Geometry: final body of the model. Coordinates: model frame, mm. Coordinates: 2 decimals unless noted, no trailing zeros. Order: outer loops, then holes, each group sorted by start corner. A loop starts at its lowest first (then second) coordinate and runs counter-clockwise, first axis right, second up. Notation, with made-up numbers: M 9.25,4 L 62.25,4 A10 ccw 62.25,20 Z; hole C -13,-31.75 d8. An arc over 180 degrees is marked long. One line per question, with ' | ' between items.
from build123d import *

# Parameters (mm, degrees)
SKETCH4_R                                         = 4.5339
SKETCH4_R_2                                       = 4.37515
CUT_EXTRUDE2_DEPTH                                = 4.064
CUT_EXTRUDE1_DEPTH                                = 4.064
CIRPATTERN1_COUNT                                 = 14
SKETCH6_R                                         = 1.5875
CUT_EXTRUDE3_DEPTH                                = 12.02520933
CUT_EXTRUDE4_DEPTH                                = 1.016
SKETCH11_R                                        = 6.731
CUT_EXTRUDE6_DEPTH                                = 2.54
SKETCH13_R                                        = 9.525
CUT_EXTRUDE7_DEPTH                                = 12.262802402
BOSS_EXTRUDE2_START                               = -4.064
SKETCH17_R                                        = 1.5875
SKETCH17_R_2                                      = 1.4732
BOSS_EXTRUDE2_DEPTH                               = 4.064
BOSS_EXTRUDE1_START                               = 2.54
SKETCH12_R                                        = 1.4732
BOSS_EXTRUDE1_DEPTH                               = 2.54
CSK_FOR_4_FLAT_HEAD_MACHINE_SCREW_100_D           = 2.9464
CSK_FOR_4_FLAT_HEAD_MACHINE_SCREW_100_CSINK_D     = 6.320409
CSK_FOR_4_FLAT_HEAD_MACHINE_SCREW_100_CSINK_ANGLE = 100


with BuildPart() as part:
    # Sketch1 → Revolve1 (revolve)
    with BuildSketch(Plane.XY, mode=Mode.PRIVATE) as revolve1_sk:
        with BuildLine():
            Line((-5.5626, 1.5875), (5.5626, 1.5875))
            Line((5.5626, 1.5875), (5.5626, 6.731))
            Line((5.5626, 6.731), (5.0419, 6.731))
            ThreePointArc((5.0419, 6.731), (4.654552953, 5.958878742), (4.5212, 5.1054))
            Line((4.5212, 5.1054), (4.5212, 4.5339))
            Line((4.5212, 4.5339), (0.4572, 4.5339))
            Line((0.4572, 4.5339), (0.4572, 5.6769))
            Line((0.4572, 5.6769), (-0.5969, 6.731))
            Line((-0.5969, 6.731), (-5.5626, 6.731))
            Line((-5.5626, 6.731), (-5.5626, 1.5875))
        make_face()
    revolve(revolve1_sk.sketch.rotate(Axis((-5.5626, 0, 0), (1, 0, 0)), 90), axis=Axis((-5.5626, 0, 0), (1, 0, 0)))

    # Sketch4 → Cut-Extrude2 (cut)
    with BuildSketch(Plane(origin=(0.4572, 0, 0), x_dir=(0, 0, -1), z_dir=(1, 0, 0))):
        Circle(SKETCH4_R)
        Circle(SKETCH4_R_2, mode=Mode.SUBTRACT)
    extrude(amount=CUT_EXTRUDE2_DEPTH, mode=Mode.SUBTRACT)

    # Sketch3 → Cut-Extrude1 (cut)
    with BuildSketch(Plane(origin=(0.4572, 0, 0), x_dir=(0, 0, -1), z_dir=(1, 0, 0))):
        with BuildLine():
            Line((-0.641613493, 4.327848154), (-0.345249615, 3.692293767))
            Line((-0.345249615, 3.692293767), (0.345249615, 3.692293767))
            Line((0.345249615, 3.692293767), (0.641613493, 4.327848154))
            ThreePointArc((0.641613493, 4.327848154), (0, 4.37515), (-0.641613493, 4.327848154))
        make_face()
    cut_extrude1 = extrude(amount=CUT_EXTRUDE1_DEPTH, mode=Mode.SUBTRACT)

    # CirPattern1: Cut-Extrude1 ×14 about axis
    cirpattern1_axis = Axis((0, 0, 0), (1, 0, 0))
    for i in range(1, CIRPATTERN1_COUNT):
        add(cut_extrude1.rotate(cirpattern1_axis, i * 360 / CIRPATTERN1_COUNT), mode=Mode.SUBTRACT)

    # Sketch6 → Cut-Extrude3 (cut, through all)
    with BuildSketch(Plane(origin=(0, 0, 0), x_dir=(1, 0, 0), z_dir=(0, 1, 0))):
        with Locations(Location((-2.5527, 0, 0), (0, 0, 90))):
            Circle(SKETCH6_R)
    extrude(amount=CUT_EXTRUDE3_DEPTH, mode=Mode.SUBTRACT)

    # Sketch11 → Cut-Extrude6 (cut)
    with BuildSketch(Plane.ZY.offset(-4.5212)):
        Circle(SKETCH11_R)
    extrude(amount=-CUT_EXTRUDE6_DEPTH, mode=Mode.SUBTRACT)


with BuildPart() as body_2:
    # Sketch7 → Revolve2 (revolve)
    with BuildSketch(Plane.XY, mode=Mode.PRIVATE) as revolve2_sk:
        Polygon((-3.7211, 6.731), (-2.5527, 6.731), (-2.5527, 1.9685), (-3.7211, 1.9685), (-3.9751, 2.2225), (-3.9751, 6.477), align=None)
    revolve(revolve2_sk.sketch.rotate(Axis((-2.5527, 1.9685, 0), (0, 1, 0)), 270), axis=Axis((-2.5527, 1.9685, 0), (0, 1, 0)))

    # Sketch8 → Cut-Extrude4 (cut)
    with BuildSketch(Plane(origin=(0, 6.731, 0), x_dir=(1, 0, 0), z_dir=(0, 1, 0))):
        Polygon((-2.5527, 0.821223023), (-3.2639, 0.410611511), (-3.2639, -0.410611511), (-2.5527, -0.821223023), (-1.8415, -0.410611511), (-1.8415, 0.410611511), align=None)
    extrude(amount=-CUT_EXTRUDE4_DEPTH, mode=Mode.SUBTRACT)


with BuildPart() as cut_extrude7_tool:
    # Sketch13 → Cut-Extrude7 (new, through all)
    with BuildSketch(Plane(origin=(0.4572, 0, 0), x_dir=(0, 0, -1), z_dir=(1, 0, 0))):
        Circle(SKETCH13_R)
    extrude(amount=-CUT_EXTRUDE7_DEPTH)


with BuildPart() as part_1:
    add(part.part)

    # Cut-Extrude7: cut by cut_extrude7_tool
    add(cut_extrude7_tool.part, mode=Mode.SUBTRACT)

    # Sketch17 → Boss-Extrude2 (add)
    with BuildSketch(Plane.ZY.offset(-0.4572).offset(BOSS_EXTRUDE2_START)):
        Circle(SKETCH17_R)
        Circle(SKETCH17_R_2, mode=Mode.SUBTRACT)
    extrude(amount=BOSS_EXTRUDE2_DEPTH)

    # Sketch12 → Boss-Extrude1 (add)
    with BuildSketch(Plane(origin=(4.5212, 0, 0), x_dir=(0, 0, -1), z_dir=(1, 0, 0)).offset(BOSS_EXTRUDE1_START)):
        with BuildLine():
            Line((6.35, 0), (6.35, -44.45))
            Line((6.35, -44.45), (-6.35, -44.45))
            Line((-6.35, -44.45), (-6.35, 0))
            ThreePointArc((-6.35, 0), (0, 6.35), (6.35, 0))
        make_face()
        with Locations(Location((0, 0, 0), (0, 0, 180))):
            Circle(SKETCH12_R, mode=Mode.SUBTRACT)
    extrude(amount=-BOSS_EXTRUDE1_DEPTH)

    # CSK for #4 Flat Head Machine Screw (100)1 (through all)
    with Locations(Plane(origin=(7.0612, 0, 0), x_dir=(0, 0, -1), z_dir=(1, 0, 0))):
        with Locations((0, -28.575), (0, -38.1)):
            CounterSinkHole(CSK_FOR_4_FLAT_HEAD_MACHINE_SCREW_100_D / 2, CSK_FOR_4_FLAT_HEAD_MACHINE_SCREW_100_CSINK_D / 2, counter_sink_angle=CSK_FOR_4_FLAT_HEAD_MACHINE_SCREW_100_CSINK_ANGLE)


with BuildPart() as body_2_1:
    add(body_2.part)

    # Cut-Extrude7: cut by cut_extrude7_tool
    add(cut_extrude7_tool.part, mode=Mode.SUBTRACT)


solid = part_1.part
1. Pin query (flat end, axial travel): P1, Ø6.5, axis at y = -15, z = -1.5, coming from the -X side; P2, Ø0.6, axis at x = 2.5, z = 0, coming from the -Y side; P3, Ø1.5, axis at x = 5.5, y = 1, coming from the +Z side. Return the tip coordinate at first contact, or that it passes through.
Response values:
P1: stops at x = 4.52 | P2: stops at y = -3.69 | P3: stops at z = 6.35
2. Section A-A, the plane y = -38.1. Output: boundary loops of the cut face in (x, z).
Response values:
outline: M 4.52,-6.35 L 7.06,-6.35 L 7.06,-3.16 L 5.65,-1.47 L 4.52,-1.47 Z; M 4.52,1.47 L 5.65,1.47 L 7.06,3.16 L 7.06,6.35 L 4.52,6.35 Z
3. Material intervals for line 1 (Y direction, x = 5.2, z = 0); line 2 (Z direction, x = 5.35, y = -38.1); line 3 (Y direction, x = 5.5, z = 0.5), sorted ascending. Write a range as [from, to].
Response values:
line 1: y = [-44.45, -39.57], [-36.63, -30.05], [-27.1, -1.47], [1.47, 6.35] | line 2: z = [-6.35, -1.47], [1.47, 6.35] | line 3: y = [-44.45, -39.49], [-36.71, -29.96], [-27.19, -1.39], [1.39, 6.33]
4. Draft query along Y for faces 1 (the face through (6, -44.45, 0)), 2 (the face through (5.08, -36.64, -0.19)), 3 (the face through (0.457, 0, 2)), 4 (the face through (5.076, -27.114, -0.192)). Return one class per face: pulls with the +Y half, pulls with the -Y half, needs draft (parallel to the pull), parting line crosses it, or undercut.
Response values:
face 1: pulls with the -Y half | face 2: undercut | face 3: needs draft | face 4: undercut
5. Section B-B, the plane y = -9. Output: boundary loops of the cut face in (x, z).
Response values:
outline: M 4.52,-6.35 L 7.06,-6.35 L 7.06,6.35 L 4.52,6.35 Z
